```python
from build123d import *

# Parameters (mm, degrees)
F0_W = 30
F0_H = 150
F4_D = 12


with BuildPart() as f2:
    # F2: sweep along a path in F1
    with BuildLine(Plane.YZ) as f2_path:
        Line((0, 0), (-150, 0))
    # F0 (on Front) → F2 (sweep)
    with BuildSketch(Plane.XZ):
        with Locations((-15, 75)):
            Rectangle(F0_W, F0_H)
    sweep(path=f2_path.line)

    # F4 (through all)
    with Locations(Plane.YZ):
        with Locations((-75, 75)):
            Hole(F4_D / 2)


solid = f2.part
```
Geometry: final body of the model. Coordinates: model frame, mm. Give positions to 0.01 mm unless a question says otherwise; leave off trailing zeros. Write each loop counter-clockwise with the first axis right and the second up, starting at its lowest first coordinate (ties: lowest second). Pieces come first, ordered by that corner, then holes.
1. Pin query (flat end, axial travel): P1, Ø11, axis at y = -75, z = 75, coming from the -X side. Return the tip coordinate at first contact, or that it passes through.
2. Line query: probe 1 along Y at (x, z) = (-3.5, 74.5); probe 2 along Z at (x, y) = (-10.25, -75). Output: solid intervals per line, ascending.
3. Draft query along Z for faces 1 (the flat face through (-15, -76, 150)), 2 (the flat face through (-30, -76, 59)), 3 (the cylindrical face through (-15.21, -70.58, 79.06)). Return one class per face: released by +Z, released by -Z, zero draft, split by the parting line, or undercut.
4. Section query A-A, the plane y = -75. Return loops of the section in (x, z).
5. Section query B-B, the plane z = 75. Return loops of the section in (x, y), then the cut area to 3 significant figures.
Computed:
1. P1: passes through
2. probe 1: y = -150 to -80.98, -69.02 to 0
2. probe 2: z = 0 to 69, 81 to 150
3. face 1: released by +Z
3. face 2: zero draft
3. face 3: undercut
4. outline: (-30, 0) - (0, 0) - (0, 69) - (-30, 69) - close; (-30, 81) - (0, 81) - (0, 150) - (-30, 150) - close
5. outline: (-30, -150) - (0, -150) - (0, -81) - (-30, -81) - close; (-30, -69) - (0, -69) - (0, 0) - (-30, 0) - close
5. area: 4,140 mm2
